CAD build for the part. Positions are in the model's coordinates, mm. A direction names the side the tool comes from. Give positions to 0.01 mm unless a question says otherwise; leave off trailing zeros. Write each loop counter-clockwise with the first axis right and the second up, starting at its lowest first coordinate (ties: lowest second). Pieces come first, ordered by that corner, then holes. Notation, with made-up numbers: (-4, 16) - (47, 16) arc R10 cw to (47, 35) - close; hole circle Ø6 at (51.5, 29.25). An arc over 180 degrees is marked (long way). Answer as a JSON object with one key per item and string values.
from build123d import *

# Parameters (mm, degrees)
POCKET_DEPTH    = 3
POCKET_FACE18_R = 2.5
POCKET001_DEPTH = 10


with BuildPart() as part:
    # Sketch → Revolution (revolve)
    with BuildSketch(Plane.XZ):
        Polygon((0, 50), (5, 50), (5, 45), (2.5, 45), (2.5, 0), (0, 0), align=None)
    revolve(axis=Axis((0, 0, 0), (0, 0, 1)))

    # Sketch001 (on Face1 of Revolution) → Pocket (cut)
    with BuildSketch(Plane(origin=(0, 0, 50), x_dir=(-1, 0, 0), z_dir=(0, 0, 1))):
        Polygon((-3.5, 0.5), (-0.5, 0.5), (-0.5, 3.5), (0.5, 3.5), (0.5, 0.5), (3.5, 0.5), (3.5, -0.5), (0.5, -0.5), (0.5, -3.5), (-0.5, -3.5), (-0.5, -0.5), (-3.5, -0.5), align=None)
    extrude(amount=-POCKET_DEPTH, mode=Mode.SUBTRACT)

    # Pocket Face18 → Pocket001 (cut)
    with BuildSketch(Plane(origin=(0, 0, 0), x_dir=(0, -1, 0), z_dir=(0, 0, -1))):
        Circle(POCKET_FACE18_R)
    extrude(amount=-POCKET001_DEPTH, mode=Mode.SUBTRACT)


solid = part.part
Item 1: Which spindle directions (+Z, -Z, +X, -X, +Y, -Y) get a long thin tool onto all of the face, cutting with end or side? Do faces 4 (the cylindrical face through (-1.08, -4.88, 47.46)), 5 (the flat face through (0.5, 2, 49)). Say none if no direction does.
Entries:
{"face 4": "+Z, -Z", "face 5": "+Z"}
Item 2: Cut at C-C (z = 46.5). Give the cut face in (x, y).
Entries:
{"outline": "circle Ø10 at (0, 0)"}
Item 3: Cut at A-A (y = 0). Give the cut face in (x, z).
Entries:
{"outline": "(-5, 45) - (-2.5, 45) - (-2.5, 10) - (2.5, 10) - (2.5, 45) - (5, 45) - (5, 50) - (3.5, 50) - (3.5, 47) - (-3.5, 47) - (-3.5, 50) - (-5, 50) - close"}
Item 4: Flat gauge pins, fed straight in: P1, Ø3.5, axis at y = -2, z = 49, coming from the +X side; P2, Ø0.9, axis at x = 2.5, z = 48.5, coming from the +Y side; P3, Ø6, axis at y = -4, z = 42.5, coming from the +X side; P4, Ø3.5, axis at x = -1.5, z = 49, coming from the -Y side. Where does each tip first touch, or does it go through?
Entries:
{"P1": "x = 4.99", "P2": "y = 4.56", "P3": "x = 4.42", "P4": "y = -5"}
Item 5: Mould opens along Y. For faces 1 (the flat face through (2, -2, 45)), 2 (the flat face through (0, 3.5, 49)), 3 (the cylindrical face through (-0.54, -2.44, 27.26)) say: +Y half, -Y half, draft (parallel to the pull), parting line (faces both ways), or undercut.
Entries:
{"face 1": "draft", "face 2": "undercut", "face 3": "parting line"}
Item 6: Probe line 1 (Z direction, x = 2.5, y = 2.25); line 2 (Z direction, x = 1.5, y = 0); line 3 (X direction, y = 0.25, z = 32). List the from-to ranges inside material, lowest first. Write a range as from..to.
Entries:
{"line 1": "45..50", "line 2": "10..47", "line 3": "-2.49..2.49"}
Item 7: Cut at D-D (x = 4). Give the cut face in (y, z), and give its area (3 significant figures).
Entries:
{"outline": "(-3, 45) - (3, 45) - (3, 50) - (-3, 50) - close", "area": "30.0 mm2"}
